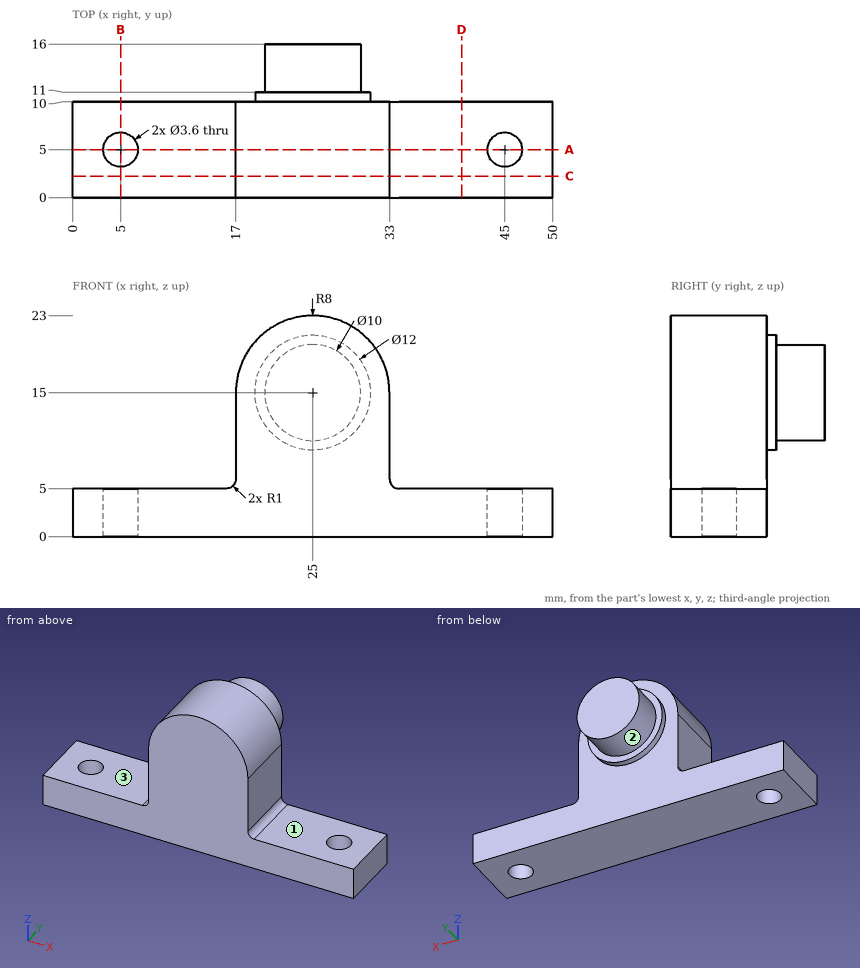
Answer from the drawing. Dimensions are ordinates in mm from the lowest x, y and z of the part. A direction names the side the tool comes from. Round coordinates to 2 decimals unless told otherwise and drop trailing zeros. Loops run counter-clockwise (first coordinate to the right, second up) from the corner with the lowest first, then second, coordinate; pieces in that order, holes last.
Q1. Section D-D on x = 40.5 is taken. Write down the section's boundary in (y, z).
Q2. Section C-C on y = 2.25 is taken. Write down the section's boundary in (x, z).
Q3. Consider probe 1 along Y at (x, z) = (5, 3.4); probe 2 along Z at (x, y) = (11, 4); probe 3 along Y at (x, z) = (29, 6.5). Determine where each line is inside the solid, lowest interval first.
Q4. Which of the six approach directions +Z, -Z, +X, -X, +Y, -Y give full straight-line access (tool end or side, diameter ignored) to the marked faces 1, 2 and 3?
Q5. Section B-B on x = 5 is taken. Write down the section's boundary in (y, z), and give its area (3 significant figures).
Q6. Each of these flat-tipped pins is pushed along its axis until it touches: pin 1 (4 mm diameter, centred on x = 32.5, z = 3.5, fed in from +Y); pin 2 (4.5 mm diameter, centred on y = 3, z = 11, fed in from -X); pin 3 (6 mm diameter, centred on x = 5, y = 5, fed in from +Z). Where does it stop, or does it pass through?
Q7. Section A-A on y = 5 is taken. Write down the section's boundary in (x, z).
Output:
1. outline: (0, 0) - (10, 0) - (10, 5) - (0, 5) - close
2. outline: (0, 0) - (50, 0) - (50, 5) - (34, 5) arc R1 cw to (33, 6) - (33, 15) arc R8 ccw to (17, 15) - (17, 6) arc R1 cw to (16, 5) - (0, 5) - close
3. probe 1: y = 0 to 3.2, 6.8 to 10
3. probe 2: z = 0 to 5
3. probe 3: y = 0 to 10
4. face 1: +Z, +X, +Y, -Y
4. face 2: +Y
4. face 3: +Z, -X, +Y, -Y
5. outline: (0, 0) - (3.2, 0) - (3.2, 5) - (0, 5) - close; (6.8, 0) - (10, 0) - (10, 5) - (6.8, 5) - close
5. area: 32.0 mm2
6. pin 1: stops at y = 10
6. pin 2: stops at x = 17
6. pin 3: stops at z = 5
7. outline: (0, 0) - (3.2, 0) - (3.2, 5) - (0, 5) - close; (6.8, 0) - (43.2, 0) - (43.2, 5) - (34, 5) arc R1 cw to (33, 6) - (33, 15) arc R8 ccw to (17, 15) - (17, 6) arc R1 cw to (16, 5) - (6.8, 5) - close; (46.8, 0) - (50, 0) - (50, 5) - (46.8, 5) - close
